Part model, mm, in its own coordinate system. Coordinates: 2 decimals unless noted, no trailing zeros. Order: outer loops, then holes, each group sorted by start corner. A loop starts at its lowest first (then second) coordinate and runs counter-clockwise, first axis right, second up.
1) Cut at B-B (z = 0). List the corners of the cut face in (x, y), and give its area (3 significant figures).
2) Mould opens along X. For faces 1 (the flat face through (-5, 0, 4.4)), 2 (the cylindrical face through (2.703, 5.923, 8.584)), 3 (the cylindrical face through (1.802, 5.923, 5.723)) say: +X half, -X half, draft (parallel to the pull), parting line (faces both ways), or undercut.
3) Cut at C-C (y = 2). List the corners of the cut face in (x, z).
4) Wall check: L1, parallel to X at y = 8.25, z = 0; L2, parallel to Z at x = -0.5, y = 10.75; L3, parallel to X at y = 1, z = 4.25. Give the ranges that are in metal, low to high.
5) Pin check, flat tips, straight feed: pin 1 Ø2 at (y, z) = (2, -6.5) entering from -X; pin 2 Ø1.5 at (x, y) = (4, 9) entering from -Z; pin 3 Ø7 at (x, z) = (0, 0) entering from -Y; pin 4 Ø1 at (y, z) = (8, 7) entering from -X. Stop position of each tip, or through.
6) Cut at A-A (x = 0). List the corners of the cut face in (y, z).
```python
from build123d import *

# Parameters (mm, degrees)
ESQUISSE1_R        = 9
ESQUISSE1_R_2      = 6
BOSS_EXTRU_1_DEPTH = 12
CHANFREIN1_SIZE    = 0.5


with BuildPart() as part:
    # Esquisse1 → Boss.-Extru.1 (new body)
    with BuildSketch(Plane(origin=(0, 0, 0), x_dir=(1, 0, 0), z_dir=(0, 1, 0))):
        with Locations(Location((0, 0, 0), (0, 0, 270))):  # turned: the seam where the file's is
            Circle(ESQUISSE1_R)
        with Locations(Location((0, 0, 0), (0, 0, 270))):  # turned: the seam where the file's is
            Circle(ESQUISSE1_R_2, mode=Mode.SUBTRACT)
    extrude(amount=BOSS_EXTRU_1_DEPTH)

    # Chanfrein1
    chanfrein1_edges = [part.edges().sort_by_distance(p)[0] for p in [
        (0, 0, -9),
        (0, 12, -9),
        (0, 0, -6),
        (0, 12, -6),
    ]]
    chamfer(chanfrein1_edges, length=CHANFREIN1_SIZE)


solid = part.part
```
Geometry check:
1. outline: (-9, 0.5) - (-8.5, 0) - (-6.5, 0) - (-6, 0.5) - (-6, 11.5) - (-6.5, 12) - (-8.5, 12) - (-9, 11.5) - close; (6, 0.5) - (6.5, 0) - (8.5, 0) - (9, 0.5) - (9, 11.5) - (8.5, 12) - (6.5, 12) - (6, 11.5) - close
1. area: 71.0 mm2
2. face 1: draft
2. face 2: parting line
2. face 3: undercut
3. outline: circle Ø18 at (0, 0); hole circle Ø12 at (0, 0)
4. L1: x = -9 to -6, 6 to 9
4. L2: z = -8.99 to -5.98, 5.98 to 8.99
4. L3: x = -7.93 to -4.24, 4.24 to 7.93
5. pin 1: stops at x = -7.12
5. pin 2: stops at z = -8.39
5. pin 3: passes through
5. pin 4: stops at x = -6.22
6. outline: (0, -8.5) - (0.5, -9) - (11.5, -9) - (12, -8.5) - (12, -6.5) - (11.5, -6) - (0.5, -6) - (0, -6.5) - close; (0, 6.5) - (0.5, 6) - (11.5, 6) - (12, 6.5) - (12, 8.5) - (11.5, 9) - (0.5, 9) - (0, 8.5) - close
